For this review, use the dimensioned drawing (mm, ordinates from the lowest corner) and the shaded views. Give positions to 0.01 mm unless a question says otherwise; leave off trailing zeros. Loops run counter-clockwise (first coordinate to the right, second up) from the corner with the lowest first, then second, coordinate; pieces in that order, holes last. Notation, with made-up numbers: (2, 61.5) -> (47, 61.5) arc R11 cw to (47, 65.5) -> close; hole circle Ø8 at (82, -24.75). An arc over 180 degrees is marked (long way). Write each question's results on one line, items separated by ' | '. Start each with the question number.
Q1. We need section B-B (x = 30.5). Write out the cut boundary in (y, z), plus the area to 3 significant figures.
Q2. Wall thickness on L1, parallel to Y at x = 5.5, z = 1.6; L2, parallel to Y at x = 56.5, z = 1.45; L3, parallel to X at y = 27, z = 2.05: over which ranges is each line inside the solid? List them lowest first. Write a range as [from, to].
Q3. Insertion check: pin 1 Ø5.5 at (x, y) = (90.5, 29.5) entering from -Z. The pin has a flat end and moves straight along its axis. Give the tip position at first contact, or say it passes through.
Q4. We need section A-A (z = 1.4). Give the number of separate pieces and of enclosed holes in the cut face, plus the area to 3 significant figures.
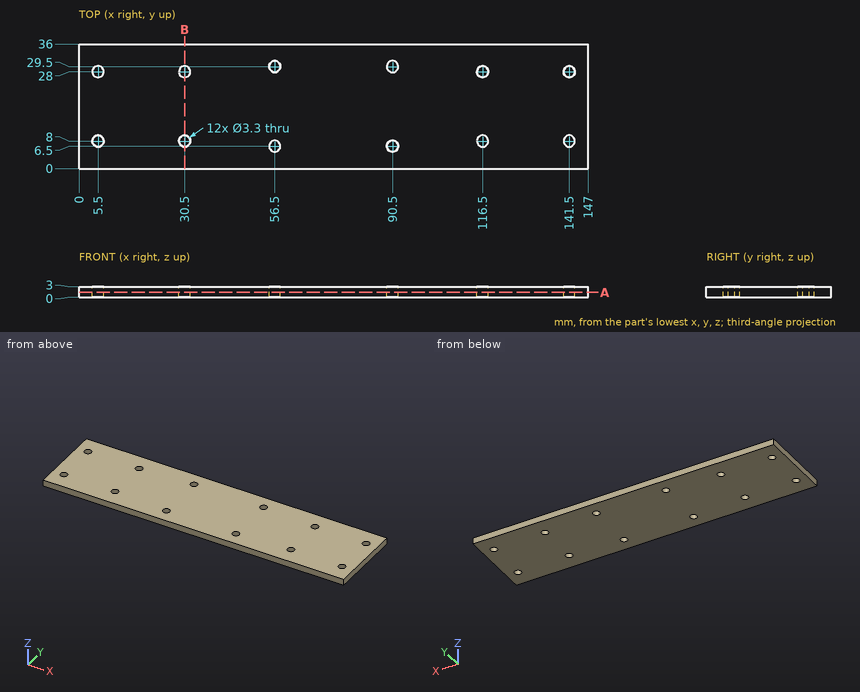
Output:
1) outline: (0, 0) -> (6.35, 0) -> (6.35, 3) -> (0, 3) -> close; (9.65, 0) -> (26.35, 0) -> (26.35, 3) -> (9.65, 3) -> close; (29.65, 0) -> (36, 0) -> (36, 3) -> (29.65, 3) -> close | area: 88.2 mm2
2) L1: [0, 6.35], [9.65, 26.35], [29.65, 36] | L2: [0, 4.85], [8.15, 27.85], [31.15, 36] | L3: [0, 4.19], [6.81, 29.19], [31.81, 115.19], [117.81, 140.19], [142.81, 147]
3) pin 1: z = 0
4) separate pieces: 1 | enclosed holes: 12 | area: 5,190 mm2
